Verification items for the finished model (mm, model axes). A direction names the side the tool comes from. Coordinates: 2 decimals unless noted, no trailing zeros. Order: outer loops, then holes, each group sorted by start corner. A loop starts at its lowest first (then second) coordinate and runs counter-clockwise, first axis right, second up. Notation, with made-up numbers: M 75,62 L 97,62 A26 ccw 97,91 Z; hole C 36,-30.5 d6. An arc over 180 degrees is marked long. Return JSON: item names as keys, results as strings.
```python
from build123d import *

# Parameters (mm, degrees)
SKETCH_1_R          = 14
SKETCH_1_R_2        = 8.5
EXTRUDE_1_DEPTH     = 5
SKETCH_2_R          = 16.127190563
SKETCH_2_R_2        = 13
CUT_EXTRUDE_1_DEPTH = 3.9
CHAMFER_1_SIZE      = 0.3


with BuildPart() as part:
    # 草图1 → 凸台-拉伸1 (new body)
    with BuildSketch(Plane(origin=(0, 0, 0), x_dir=(0, 0, -1), z_dir=(1, 0, 0))):
        Circle(SKETCH_1_R)
        Circle(SKETCH_1_R_2, mode=Mode.SUBTRACT)
    extrude(amount=EXTRUDE_1_DEPTH)

    # 草图2 → 切除-拉伸1 (cut)
    with BuildSketch(Plane(origin=(5, 0, 0), x_dir=(0, 0, -1), z_dir=(1, 0, 0))):
        Circle(SKETCH_2_R)
        Circle(SKETCH_2_R_2, mode=Mode.SUBTRACT)
    extrude(amount=-CUT_EXTRUDE_1_DEPTH, mode=Mode.SUBTRACT)

    # 倒角1
    chamfer_1_edges = [part.edges().sort_by_distance(p)[0] for p in [
        (5, 0, 13),
        (0, 0, 14),
        (0, 0, 8.5),
        (5, 0, 8.5),
    ]]
    chamfer(chamfer_1_edges, length=CHAMFER_1_SIZE)


solid = part.part
```
Q1. Material ranges on line 1 along Y through (x, z) = (3.85, 0); line 2 along Y through (x, z) = (0.55, 0.25); line 3 along Z through (x, y) = (2.9, 7.25), recorded low to high.
Values:
{"line 1": "-13 to -8.5, 8.5 to 13", "line 2": "-14 to -8.5, 8.5 to 14", "line 3": "-10.79 to -4.44, 4.44 to 10.79"}
Q2. Cross-section at A-A, the plane y = 0. Record the boundary of the cut face in (x, z), and give its area (3 significant figures).
Values:
{"outline": "M 0,-13.7 L 0.3,-14 L 1.1,-14 L 1.1,-13 L 4.7,-13 L 5,-12.7 L 5,-8.8 L 4.7,-8.5 L 0.3,-8.5 L 0,-8.8 Z; M 0,8.8 L 0.3,8.5 L 4.7,8.5 L 5,8.8 L 5,12.7 L 4.7,13 L 1.1,13 L 1.1,14 L 0.3,14 L 0,13.7 Z", "area": "46.8 mm^2"}
Q3. Go/stop test with flat-tipped pins: pin 1 (2 mm diameter, centred on x = 2, z = -6.5, fed in from -Y); pin 2 (1.5 mm diameter, centred on x = 1, y = 6, fed in from +Z); pin 3 (2 mm diameter, centred on x = 1.5, z = -2, fed in from -Y). Record where each tip stops, or that it passes through.
Values:
{"pin 1": "y = -12.62", "pin 2": "z = 12.98", "pin 3": "y = -13.96"}
Q4. Cross-section at C-C, the plane x = 2.05. Record the boundary of the cut face in (y, z), and give its area (3 significant figures).
Values:
{"outline": "C 0,0 d26; hole C 0,0 d17", "area": "304 mm^2"}
Q5. Tool access check on faces 1 (the face through (1.1, -9.3, -9.3)), 2 (the face through (5, 9, -3)). Record the directions out of +Z, -Z, +X, -X, +Y, -Y that give a thin tool (end or side, any length) a straight path to the whole face; none if there is none.
Values:
{"face 1": "+X", "face 2": "+Z, -Z, +X, +Y, -Y"}
Q6. Draft check along Y on faces 3 (the face through (0.694, -5.362, -12.932)), 4 (the face through (0, -9, 0)), 5 (the face through (2.469, 7.167, -4.57)). Enter one of: pulls with the +Y half, pulls with the -Y half, needs draft (parallel to the pull), parting line crosses it, or undercut.
Values:
{"face 3": "parting line crosses it", "face 4": "needs draft", "face 5": "undercut"}
